Model file for the job. Use its own axes, mm. A direction names the side the tool comes from. Round coordinates to 2 decimals unless told otherwise and drop trailing zeros. Write each loop counter-clockwise with the first axis right and the second up, starting at its lowest first coordinate (ties: lowest second). Pieces come first, ordered by that corner, then holes. Notation, with made-up numbers: (-34.75, -21.75) - (5.25, -21.75) arc R20 cw to (5.25, -11.75) - close; hole circle Ø1 at (-25.5, 67). An arc over 180 degrees is marked (long way). One line per item, written item: value.
Autodesk Inventor part; units mm, degrees
ref_plane "YZ Plane" through (0, 0, 0) normal (1, 0, 0) x (0, 1, 0)
ref_plane "XZ Plane" through (0, 0, 0) normal (0, 1, 0) x (-1, 0, 0)
ref_plane "XY Plane" through (0, 0, 0) normal (0, 0, 1) x (1, 0, 0)
sketch "Sketch1" plane through (0, 0, 0) normal (0, 1, 0) x (-1, 0, 0)
  line L0 (-20, -50) -> (20, -50)
  line L1 (20, -50) -> (20, 50)
  line L2 (20, 50) -> (-20, 50)
  line L3 (-20, 50) -> (-20, -50)
  line L4 (-20, -50) -> (20, 50) construction
  line L5 (20, -50) -> (-20, 50) construction
  point P0 (0, 0)
  dimension "d2" = 40
  dimension "d3" = 100
extrude "Extrusion1" add sketch "Sketch1" along normal blind 5
sketch "Sketch2" plane through (0, 5, 0) normal (0, 1, 0) x (1, 0, 0)
  line L0 (-20, 50) -> (-20, -50)
  line L1 (-20, -50) -> (20, -50)
  line L2 (20, -50) -> (20, 50)
  line L3 (20, 50) -> (-20, 50)
  line L4 (17, 47) -> (-17, 47)
  line L5 (-17, 47) -> (-17, -47)
  line L6 (-17, -47) -> (17, -47)
  line L7 (17, -47) -> (17, 47)
  line L8 (17, 47) -> (-17, -47) construction
  line L9 (-17, 47) -> (17, -47) construction
  line L10 (15, 45) -> (-15, 45)
  line L11 (-15, 45) -> (-15, -45)
  line L12 (-15, -45) -> (15, -45)
  line L13 (15, -45) -> (15, 45)
  line L14 (15, 45) -> (-15, -45) construction
  line L15 (-15, 45) -> (15, -45) construction
  point P0 (0, 0)
  dimension "d6" = 3
  dimension "d7" = 2
  dimension "d52" = 3
  dimension "d53" = 2
extrude "Extrusion2" add sketch "Sketch2" along normal blind 40 contours L7 L6 L5 L4
fillet "Fillet1" radius 1 1 edges at (20, 2.5, 50)
fillet "Fillet2" radius 1 1 edges at (20, 2.5, -50)
fillet "Fillet3" radius 1 1 edges at (-20, 2.5, 50)
fillet "Fillet4" radius 1 1 edges at (-20, 2.5, -50)
fillet "Fillet5" radius 1 1 edges at (-17, 25, 47)
fillet "Fillet6" radius 1 1 edges at (17, 25, 47)
fillet "Fillet7" radius 1 1 edges at (17, 25, -47)
fillet "Fillet8" radius 1 1 edges at (-17, 25, -47)
sketch "Sketch3" plane through (0, 45, 0) normal (0, 1, 0) x (1, 0, 0)
  arc A0 (-16, 47) -> (-17, 46) centre (-16, 46) ccw
  line L0 (-17, 46) -> (-17, -46)
  arc A1 (-17, -46) -> (-16, -47) centre (-16, -46) ccw
  line L1 (-16, -47) -> (16, -47)
  arc A2 (16, -47) -> (17, -46) centre (16, -46) ccw
  line L2 (17, -46) -> (17, 46)
  arc A3 (17, 46) -> (16, 47) centre (16, 46) ccw
  line L3 (16, 47) -> (-16, 47)
  line L4 (15, 45) -> (15, -45)
  line L5 (15, -45) -> (-15, -45)
  line L6 (-15, -45) -> (-15, 45)
  line L7 (-15, 45) -> (15, 45)
  line L8 (-16.5, -40) -> (-15.5, -40)
  line L9 (-15.5, -40) -> (-15.5, -20)
  line L10 (-15.5, -20) -> (-16.5, -20)
  line L11 (-16.5, -20) -> (-16.5, -40)
  line L12 (-16.5, 40) -> (-15.5, 40)
  line L13 (-15.5, 40) -> (-15.5, 20)
  line L14 (-15.5, 20) -> (-16.5, 20)
  line L15 (-16.5, 20) -> (-16.5, 40)
  line L16 (-10, 46.5) -> (10, 46.5)
  line L17 (10, 46.5) -> (10, 45.5)
  line L18 (10, 45.5) -> (-10, 45.5)
  line L19 (-10, 45.5) -> (-10, 46.5)
  line L20 (10, 46.5) -> (-10, 46.5)
  line L21 (-10, 46.5) -> (-10, 45.5)
  line L22 (-10, 45.5) -> (10, 45.5)
  line L23 (10, 45.5) -> (10, 46.5)
  line L24 (15.5, 40) -> (16.5, 40)
  line L25 (16.5, 40) -> (16.5, 20)
  line L26 (16.5, 20) -> (15.5, 20)
  line L27 (15.5, 20) -> (15.5, 40)
  line L28 (15.5, -40) -> (16.5, -40)
  line L29 (16.5, -40) -> (16.5, -20)
  line L30 (16.5, -20) -> (15.5, -20)
  line L31 (15.5, -20) -> (15.5, -40)
  line L32 (10, -45.5) -> (-10, -45.5)
  line L33 (-10, -45.5) -> (-10, -46.5)
  line L34 (-10, -46.5) -> (10, -46.5)
  line L35 (10, -46.5) -> (10, -45.5)
  line L36 (-10, -45.5) -> (10, -45.5)
  line L37 (10, -45.5) -> (10, -46.5)
  line L38 (10, -46.5) -> (-10, -46.5)
  line L39 (-10, -46.5) -> (-10, -45.5)
  point P0 (0, 0)
  point P1 (-16, 40)
  point P2 (-16, 20)
  point P3 (16, 40)
  dimension "d18" = 1
  dimension "d19" = 20
  dimension "d20" = 0.5
  dimension "d21" = 7
  dimension "d22" = 7
  dimension "d23" = 0.5
  dimension "d24" = 1
  dimension "d25" = 20
  dimension "d26" = 20
  dimension "d27" = 1
  dimension "d28" = 0.5
  dimension "d29" = 7
  dimension "d30" = 20
  dimension "d31" = 1
  dimension "d32" = 0.5
  dimension "d33" = 7
  dimension "d34" = 1
  dimension "d35" = 20
  dimension "d36" = 0.5
  dimension "d37" = 7
  dimension "d38" = 1
  dimension "d39" = 20
  dimension "d40" = 7
  dimension "d41" = 0.5
  dimension "d42" = 20
  dimension "d43" = 1
  dimension "d44" = 0.5
  dimension "d45" = 7
  dimension "d46" = 20
  dimension "d47" = 1
  dimension "d48" = 0.5
  dimension "d49" = 7
extrude "Extrusion3" cut sketch "Sketch3" against normal blind 1 contours L11 L10 L9 L8 | L12 L13 L14 L15 | L16 L17 L18 L19 | L24 L25 L26 L27 | L31 L30 L29 L28 | L35 L34 L33 L32
properties part number "block_main" material "PC/ABS Plastic"
1. Band-saw the part on C-C on x = -3. Write the cut outline in (y, z).
Report:
outline: (0, -50) - (5, -50) - (5, -47) - (45, -47) - (45, -46.5) - (44, -46.5) - (44, -45.5) - (45, -45.5) - (45, -45) - (5, -45) - (5, 45) - (45, 45) - (45, 45.5) - (44, 45.5) - (44, 46.5) - (45, 46.5) - (45, 47) - (5, 47) - (5, 50) - (0, 50) - close
2. Band-saw the part on B-B on z = -7.5. Write the cut outline in (x, y), plus the area to 3 significant figures.
Report:
outline: (-20, 0) - (20, 0) - (20, 5) - (17, 5) - (17, 45) - (15, 45) - (15, 5) - (-15, 5) - (-15, 45) - (-17, 45) - (-17, 5) - (-20, 5) - close
area: 360 mm²
3. Mould opens along X. For faces 1 (the face through (0, 0, 1)), 2 (the face through (0, 25, 45)), 3 (the face through (-17, 25, -1)), 4 (the face through (17, 25, 1)) say: released by +X, released by -X, zero draft, split by the parting line, or undercut.
Report:
face 1: zero draft
face 2: undercut
face 3: released by -X
face 4: released by +X
4. Tool access for faces 5 (the face through (-20, 2, -1)), 6 (the face through (0, 25, -47)), 7 (the face through (0, 2, 50)), 8 (the face through (0, 25, 47)), 9 (the face through (18, 5, 4)): list every direction of +Z, -Z, +X, -X, +Y, -Y with a clear straight run to the whole face (end or side of a thin tool).
Report:
face 5: +Z, -Z, -X, +Y, -Y
face 6: -Z, +X, -X, +Y
face 7: +Z, +X, -X, +Y, -Y
face 8: +Z, +X, -X, +Y
face 9: +Y
5. Band-saw the part on A-A on y = 26. Write the cut outline in (x, z).
Report:
outline: (-17, -46) arc R1 ccw to (-16, -47) - (16, -47) arc R1 ccw to (17, -46) - (17, 46) arc R1 ccw to (16, 47) - (-16, 47) arc R1 ccw to (-17, 46) - close; hole (-15, -45) - (15, -45) - (15, 45) - (-15, 45) - close
6. Wall check: probe 1 along X at (y, z) = (29, -19.5); probe 2 along Z at (x, y) = (11, 18); probe 3 along Y at (x, z) = (-16, -37). Give the ranges that are in metal, low to high. Write a range as [from, to].
Report:
probe 1: [-17, -15], [15, 17]
probe 2: [-47, -45], [45, 47]
probe 3: [0, 44]
7. Band-saw the part on D-D on z = 22. Write the cut outline in (x, y), plus the area to 3 significant figures.
Report:
outline: (-20, 0) - (20, 0) - (20, 5) - (17, 5) - (17, 45) - (16.5, 45) - (16.5, 44) - (15.5, 44) - (15.5, 45) - (15, 45) - (15, 5) - (-15, 5) - (-15, 45) - (-15.5, 45) - (-15.5, 44) - (-16.5, 44) - (-16.5, 45) - (-17, 45) - (-17, 5) - (-20, 5) - close
area: 358 mm²
8. Drop flat-ended pins along their axis: pin 1 (0.8 mm diameter, centred on y = 44.5, z = 46, fed in from +X); pin 2 (1.5 mm diameter, centred on x = 2, z = 10.5, fed in from +Y); pin 3 (1.1 mm diameter, centred on x = -3, y = 44.5, fed in from -Z); pin 4 (1.1 mm diameter, centred on x = 16, z = -35, fed in from +Y). Give the stop position or say it passes through.
Report:
pin 1: x = 17
pin 2: y = 5
pin 3: z = -47
pin 4: y = 45
